Autodesk Inventor part; units mm, degrees
ref_plane "YZ Plane" through (0, 0, 0) normal (1, 0, 0) x (0, 1, 0)
ref_plane "XZ Plane" through (0, 0, 0) normal (0, 1, 0) x (-1, 0, 0)
ref_plane "XY Plane" through (0, 0, 0) normal (0, 0, 1) x (1, 0, 0)
sketch "Sketch1" plane through (0, 0, 0) normal (1, 0, 0) x (0, 1, 0)
  line L0 (0, 0) -> (61, 0)
  line L1 (61, 0) -> (61, -200)
  line L2 (61, -200) -> (0, -200)
  line L3 (0, -200) -> (0, 0)
  line L4 (51.4645, -6) -> (9.5355, -6)
  circle A0 centre (30.5, -173) radius 8.625
  circle A1 centre (30.5, -123) radius 17
  circle A2 centre (30.5, -59) radius 8.625
  line L5 (55, -51.4645) -> (55, -9.5355)
  line L6 (55, -9.5355) -> (34.0355, -30.5)
  line L7 (6, -9.5355) -> (26.9645, -30.5)
  line L8 (51.4645, -6) -> (30.5, -26.9645)
  line L9 (26.9645, -30.5) -> (6, -51.4645)
  line L10 (9.5355, -6) -> (30.5, -26.9645)
  line L11 (34.0355, -30.5) -> (55, -51.4645)
  line L12 (6, -9.5355) -> (6, -51.4645)
  line L13 (51.4645, -111.0711) -> (55, -114.6066)
  line L14 (9.5355, -111.0711) -> (6, -114.6066)
  line L15 (55, -107.5355) -> (55, -65.6066)
  line L16 (26.9645, -86.5711) -> (6, -107.5355)
  line L17 (34.0355, -86.5711) -> (55, -107.5355)
  line L18 (55, -65.6066) -> (34.0355, -86.5711)
  line L19 (28, -92.6066) -> (9.5355, -111.0711)
  line L20 (6, -65.6066) -> (26.9645, -86.5711)
  line L21 (33, -92.6066) -> (51.4645, -111.0711)
  line L22 (6, -65.6066) -> (6, -107.5355)
  line L23 (40.9822, -44.5178) -> (52.9645, -56.5)
  line L24 (52.0355, -61.5) -> (33, -80.5355)
  line L25 (28, -80.5355) -> (8.9645, -61.5)
  line L26 (8.0355, -56.5) -> (28, -36.5355)
  line L27 (33, -36.5355) -> (40.9822, -44.5178)
  line L28 (33, -36.5355) -> (33, -46.7526)
  line L29 (33, -71.2474) -> (33, -80.5355)
  line L30 (28, -36.5355) -> (28, -46.7526)
  line L31 (28, -71.2474) -> (28, -80.5355)
  line L32 (18.2526, -61.5) -> (8.9645, -61.5)
  line L33 (18.2526, -56.5) -> (8.0355, -56.5)
  arc A3 (28, -46.7526) -> (18.2526, -56.5) centre (30.5, -59) ccw
  arc A4 (18.2526, -61.5) -> (28, -71.2474) centre (30.5, -59) ccw
  arc A5 (33, -71.2474) -> (42.7474, -61.5) centre (30.5, -59) ccw
  arc A6 (42.7474, -56.5) -> (33, -46.7526) centre (30.5, -59) ccw
  line L34 (52.0355, -61.5) -> (42.7474, -61.5)
  line L35 (52.9645, -56.5) -> (42.7474, -56.5)
  line L36 (10.8223, -175.5) -> (28, -192.6777)
  line L37 (50.1777, -175.5) -> (33, -192.6777)
  line L38 (38.7487, -194) -> (55, -177.7487)
  line L39 (6, -177.7487) -> (22.2513, -194)
  line L40 (9.5355, -167.1421) -> (6.1777, -170.5)
  line L41 (51.4645, -167.1421) -> (54.8223, -170.5)
  line L42 (55, -194) -> (55, -177.7487)
  line L43 (55, -163.6066) -> (55, -121.6777)
  line L44 (6, -194) -> (22.2513, -194)
  line L45 (38.7487, -194) -> (55, -194)
  line L46 (6, -121.6777) -> (6, -163.6066)
  line L47 (6, -177.7487) -> (6, -194)
  line L48 (6, -114.6066) -> (9.1371, -117.7437)
  line L49 (6, -121.6777) -> (8.5334, -124.211)
  line L50 (35.7563, -144.3629) -> (55, -163.6066)
  line L51 (55, -114.6066) -> (51.8629, -117.7437)
  line L52 (25.2437, -144.3629) -> (6, -163.6066)
  line L53 (55, -121.6777) -> (52.4666, -124.211)
  line L54 (28, -148.6777) -> (9.5355, -167.1421)
  line L55 (33, -148.6777) -> (51.4645, -167.1421)
  arc A7 (8.5334, -124.211) -> (25.2437, -144.3629) centre (30.5, -123) ccw
  arc A8 (35.7563, -144.3629) -> (52.4666, -124.211) centre (30.5, -123) ccw
  line L56 (33, -160.7526) -> (33, -148.6777)
  line L57 (33, -185.2474) -> (33, -192.6777)
  line L58 (28, -185.2474) -> (28, -192.6777)
  line L59 (42.7474, -175.5) -> (50.1777, -175.5)
  line L60 (42.7474, -170.5) -> (54.8223, -170.5)
  line L61 (18.2526, -170.5) -> (6.1777, -170.5)
  line L62 (28, -160.7526) -> (28, -148.6777)
  line L63 (18.2526, -175.5) -> (10.8223, -175.5)
  arc A9 (18.2526, -175.5) -> (28, -185.2474) centre (30.5, -173) ccw
  arc A10 (33, -185.2474) -> (42.7474, -175.5) centre (30.5, -173) ccw
  arc A11 (42.7474, -170.5) -> (33, -160.7526) centre (30.5, -173) ccw
  arc A12 (28, -160.7526) -> (18.2526, -170.5) centre (30.5, -173) ccw
  line L64 (33, -92.6066) -> (33, -101.1425)
  line L65 (28, -92.6066) -> (28, -101.1425)
  arc A13 (51.8629, -117.7437) -> (33, -101.1425) centre (30.5, -123) ccw
  arc A14 (28, -101.1425) -> (9.1371, -117.7437) centre (30.5, -123) ccw
  dimension "d0" = 61
  dimension "d1" = 200
  dimension "d49" = 17.25
  dimension "d50" = 34
  dimension "d51" = 17.25
extrude "Extrusion1" add sketch "Sketch1" along normal blind 6
sketch "Sketch2" plane through (0, 0, 0) normal (-1, 0, 0) x (0, 0, 1)
  line L0 (0, 0) -> (-200, 0)
  line L1 (-200, 61) -> (0, 61)
  line L2 (-200, 0) -> (-200, 61)
  line L3 (0, 61) -> (0, 0)
  point P0 (-197, 58)
  point P1 (-197, 3)
  point P2 (-3, 58)
  point P3 (-3, 3)
hole "Hole1" at (0, 58, -3) at (0, 58, -197) at (0, 3, -197) at (0, 3, -3) direction (1, 0, 0) diameter 3.25 depth 6 countersink diameter 5 countersink angle 90
sketch "Sketch3" plane through (6, 0, 0) normal (1, 0, 0) x (0, 0, -1)
  circle A0 centre (173, 30.5) radius 8.625
  circle A1 centre (230, 30.5) radius 2.75
  circle A2 centre (230, 30.5) radius 8.75
  line L0 (200, 0) -> (200, 61)
  line L1 (245, 30.5) -> (245, 61)
  line L2 (200, 0) -> (200, 61)
  line L3 (200, 61) -> (245, 61)
  line L4 (245, 30.5) -> (245, 0)
  line L5 (245, 0) -> (200, 0)
  point P0 (0, 0)
  dimension "d53" = 5.5
  dimension "d54" = 17.5
  dimension "d55" = 15
extrude "Extrusion2" add sketch "Sketch3" against normal blind 6 contours L0 L3 L1 L4 L5
fillet "Fillet1" radius 30.5 2 edges at (3, 61, -245) (3, 0, -245)
properties part number "Side_Piece"
The listing builds one solid part. Answer for the finished solid, in the listing's coordinates (mm). Coordinates: 2 decimals unless noted, no trailing zeros. Write each loop counter-clockwise with the first axis right and the second up, starting at its lowest first coordinate (ties: lowest second). Pieces come first, ordered by that corner, then holes. Notation, with made-up numbers: (9, -19) - (43, -19) arc R13 ccw to (43, -8) - close; hole circle Ø11 at (29, 15.25). An arc over 180 degrees is marked (long way). Return JSON: item names as keys, results as strings. Group by question number.
Q1. The part is cut by section C-C on z = -17. Write down the section's boundary in (x, y).
Q2. The part is cut by section D-D on x = 1.8. State how many separate pieces and enclosed holes the cut face has, and give its area (3 significant figures).
Q3. The part is cut by section A-A on z = -173. Write down the section's boundary in (x, y) (3 decimals).
Q4. Flat-ended cylindrical pins translate along their axes: pin 1 Ø3 at (x, y) = (5, 14) entering from -Z; pin 2 Ø3 at (x, y) = (2.5, 22.5) entering from -Z. Find the tip coordinate at first contact, or state that the pin passes through.
Q5. The part is cut by section B-B on z = -76. Write down the section's boundary in (x, y).
Q6. Find the intervals of material crossed by line 1 along Y through (x, z) = (4.9, -197) (3 decimals); line 2 along Y through (x, z) = (0.5, -84.5); line 3 along Y through (x, z) = (2.85, -21.5), in increasing order. Write a range as [from, to].
Evaluation:
{
 "1": {"outline": "(0, 0) - (6, 0) - (6, 6) - (0, 6) - close; (0, 13.46) - (6, 13.46) - (6, 20.54) - (0, 20.54) - close; (0, 40.46) - (6, 40.46) - (6, 47.54) - (0, 47.54) - close; (0, 55) - (6, 55) - (6, 61) - (0, 61) - close"},
 "2": {"separate pieces": "1", "enclosed holes": "27", "area": "8,610 mm2"},
 "3": {"outline": "(0, 0) - (6, 0) - (6, 21.875) - (0, 21.875) - close; (0, 39.125) - (6, 39.125) - (6, 61) - (0, 61) - close"},
 "4": {"pin 1": "stops at z = -241.06", "pin 2": "stops at z = -244.3"},
 "5": {"outline": "(0, 0) - (6, 0) - (6, 6) - (0, 6) - close; (0, 16.39) - (6, 16.39) - (6, 23.46) - (0, 23.46) - close; (0, 28) - (6, 28) - (6, 33) - (0, 33) - close; (0, 37.54) - (6, 37.54) - (6, 44.61) - (0, 44.61) - close; (0, 55) - (6, 55) - (6, 61) - (0, 61) - close"},
 "6": {"line 1": "y = [0, 1.375], [4.625, 56.375], [59.625, 61]", "line 2": "y = [0, 6], [24.89, 36.11], [55, 61]", "line 3": "y = [0, 6], [17.96, 25.04], [35.96, 43.04], [55, 61]"}
}
